Here's how the part is built. I have some questions about the finished solid (model axes, mm). A direction names the side the tool comes from. Give positions to 0.01 mm unless a question says otherwise; leave off trailing zeros. Loops run counter-clockwise (first coordinate to the right, second up) from the corner with the lowest first, then second, coordinate; pieces in that order, holes last. Notation, with made-up numbers: (-2, 68) - (37, 68) arc R19 ccw to (37, 73) - close; hole circle Ø3 at (-38, 7). An arc over 180 degrees is marked (long way). Return JSON: item names as keys, results as strings. Group by question number.
(1) If we section it at D-D (z = 19.5): State how many separate pieces and enclosed holes the cut face has, then the cut area to 3 significant figures.
(2) If we section it at B-B (y = 6.75): Please give me the cut outline in (x, z), then the cut area to 3 significant figures.
(3) If we section it at A-A (x = -11.25): Please give me the cut outline in (y, z) (3 decimals).
(4) I need wall thicknesses on probe 1 along X at (y, z) = (-12, 0) (3 decimals); probe 2 along Y at (x, z) = (-5.25, 6). Which ranges of each line are inside material? Lowest first, please. Write a range as [from, to].
(5) On a 3-axis mill with a long thin cutter (end or side, diameter ignored), from which of +Z, -Z, +X, -X, +Y, -Y can I reach the whole of each face in a straight line? I mean faces 1 (the flat face through (6, -3, 0)), 2 (the flat face through (11, 8.325, 0)), 3 (the flat face through (4.2, -13, 0)), 4 (the flat face through (3, 6, 0)). Say none if no direction works.
(6) If we mould it in two halves opening along X, with no side actions, what happens to faces 5 (the flat face through (-11, -8.325, 0)), 6 (the flat face through (-13, 4.2, 0)), 7 (the flat face through (-6, 3, 0))? For each: released by +X, released by -X, zero draft, split by the parting line, or undercut.
(7) If we section it at C-C (y = 2.5): Please give me the cut outline in (x, z), then the cut area to 3 significant figures.
(8) For P1, Ø5, axis at x = 0, y = 1, coming from the +Z side, with a flat end and sliding along its axis, tell me the tip position at first contact or that it passes through.
```python
from build123d import *

# Parameters (mm, degrees)
BOSS_EXTRUDE1_DEPTH = 30


with BuildPart() as part:
    # Sketch1 → Boss-Extrude1 (new body, symmetric)
    with BuildSketch(Plane.XY):
        with BuildLine():
            Line((-8.325, 12.75), (-4.2, 12.75))
            Line((-4.2, 12.75), (-4.2, 14))
            ThreePointArc((-4.2, 14), (-4.331801948, 14.318198052), (-4.65, 14.45))
            Line((-4.65, 14.45), (-4.7, 14.45))
            Line((-4.7, 14.45), (-4.7, 14.5))
            ThreePointArc((-4.7, 14.5), (-4.831801948, 14.818198052), (-5.15, 14.95))
            Line((-5.15, 14.95), (-13.2, 14.95))
            ThreePointArc((-13.2, 14.95), (-14.437436867, 14.437436867), (-14.95, 13.2))
            Line((-14.95, 13.2), (-14.95, 5.15))
            ThreePointArc((-14.95, 5.15), (-14.818198052, 4.831801948), (-14.5, 4.7))
            Line((-14.5, 4.7), (-14.45, 4.7))
            Line((-14.45, 4.7), (-14.45, 4.65))
            ThreePointArc((-14.45, 4.65), (-14.318198052, 4.331801948), (-14, 4.2))
            Line((-14, 4.2), (-12.75, 4.2))
            Line((-12.75, 4.2), (-12.75, 8.325))
            Line((-12.75, 8.325), (-10.13519336, 8.325))
            Line((-10.13519336, 8.325), (-6, 4.18980664))
            Line((-6, 4.18980664), (-6, 0.875))
            Line((-6, 0.875), (-5.5, 0))
            Line((-5.5, 0), (-6, -0.875))
            Line((-6, -0.875), (-6, -4.18980664))
            Line((-6, -4.18980664), (-10.13519336, -8.325))
            Line((-10.13519336, -8.325), (-12.75, -8.325))
            Line((-12.75, -8.325), (-12.75, -4.2))
            Line((-12.75, -4.2), (-14, -4.2))
            ThreePointArc((-14, -4.2), (-14.318198052, -4.331801948), (-14.45, -4.65))
            Line((-14.45, -4.65), (-14.45, -4.7))
            Line((-14.45, -4.7), (-14.5, -4.7))
            ThreePointArc((-14.5, -4.7), (-14.818198052, -4.831801948), (-14.95, -5.15))
            Line((-14.95, -5.15), (-14.95, -13.2))
            ThreePointArc((-14.95, -13.2), (-14.437436867, -14.437436867), (-13.2, -14.95))
            Line((-13.2, -14.95), (-5.15, -14.95))
            ThreePointArc((-5.15, -14.95), (-4.831801948, -14.818198052), (-4.7, -14.5))
            Line((-4.7, -14.5), (-4.7, -14.45))
            Line((-4.7, -14.45), (-4.65, -14.45))
            ThreePointArc((-4.65, -14.45), (-4.331801948, -14.318198052), (-4.2, -14))
            Line((-4.2, -14), (-4.2, -12.75))
            Line((-4.2, -12.75), (-8.325, -12.75))
            Line((-8.325, -12.75), (-8.325, -10.13519336))
            Line((-8.325, -10.13519336), (-4.18980664, -6))
            Line((-4.18980664, -6), (-0.875, -6))
            Line((-0.875, -6), (0, -5.5))
            Line((0, -5.5), (0.875, -6))
            Line((0.875, -6), (4.18980664, -6))
            Line((4.18980664, -6), (8.325, -10.13519336))
            Line((8.325, -10.13519336), (8.325, -12.75))
            Line((8.325, -12.75), (4.2, -12.75))
            Line((4.2, -12.75), (4.2, -14))
            ThreePointArc((4.2, -14), (4.331801948, -14.318198052), (4.65, -14.45))
            Line((4.65, -14.45), (4.7, -14.45))
            Line((4.7, -14.45), (4.7, -14.5))
            ThreePointArc((4.7, -14.5), (4.831801948, -14.818198052), (5.15, -14.95))
            Line((5.15, -14.95), (13.2, -14.95))
            ThreePointArc((13.2, -14.95), (14.437436867, -14.437436867), (14.95, -13.2))
            Line((14.95, -13.2), (14.95, -5.15))
            ThreePointArc((14.95, -5.15), (14.818198052, -4.831801948), (14.5, -4.7))
            Line((14.5, -4.7), (14.45, -4.7))
            Line((14.45, -4.7), (14.45, -4.65))
            ThreePointArc((14.45, -4.65), (14.318198052, -4.331801948), (14, -4.2))
            Line((14, -4.2), (12.75, -4.2))
            Line((12.75, -4.2), (12.75, -8.325))
            Line((12.75, -8.325), (10.13519336, -8.325))
            Line((10.13519336, -8.325), (6, -4.18980664))
            Line((6, -4.18980664), (6, -0.875))
            Line((6, -0.875), (5.5, 0))
            Line((5.5, 0), (6, 0.875))
            Line((6, 0.875), (6, 4.18980664))
            Line((6, 4.18980664), (10.134787333, 8.324593973))
            Line((10.134787333, 8.324593973), (12.75, 8.324593973))
            Line((12.75, 8.324593973), (12.75, 4.2))
            Line((12.75, 4.2), (14, 4.2))
            ThreePointArc((14, 4.2), (14.318198052, 4.331801948), (14.45, 4.65))
            Line((14.45, 4.65), (14.45, 4.7))
            Line((14.45, 4.7), (14.5, 4.7))
            ThreePointArc((14.5, 4.7), (14.818198052, 4.831801948), (14.95, 5.15))
            Line((14.95, 5.15), (14.95, 13.2))
            ThreePointArc((14.95, 13.2), (14.437436867, 14.437436867), (13.2, 14.95))
            Line((13.2, 14.95), (5.15, 14.95))
            ThreePointArc((5.15, 14.95), (4.831801948, 14.818198052), (4.7, 14.5))
            Line((4.7, 14.5), (4.7, 14.45))
            Line((4.7, 14.45), (4.65, 14.45))
            ThreePointArc((4.65, 14.45), (4.331801948, 14.318198052), (4.2, 14))
            Line((4.2, 14), (4.2, 12.75))
            Line((4.2, 12.75), (8.324593973, 12.75))
            Line((8.324593973, 12.75), (8.324593973, 10.134787333))
            Line((8.324593973, 10.134787333), (4.18980664, 6))
            Line((4.18980664, 6), (0.875, 6))
            Line((0.875, 6), (0, 5.5))
            Line((0, 5.5), (-0.875, 6))
            Line((-0.875, 6), (-4.18980664, 6))
            Line((-4.18980664, 6), (-8.325, 10.13519336))
            Line((-8.325, 10.13519336), (-8.325, 12.75))
        make_face()
        with BuildLine():
            Line((-4.478803313, -3.194699355), (-3.226318161, -1.597144679))
            ThreePointArc((-3.226318161, -1.597144679), (-3.6, 0), (-3.226318161, 1.597144679))
            Line((-3.226318161, 1.597144679), (-4.478803313, 3.194699355))
            ThreePointArc((-4.478803313, 3.194699355), (-3.890101739, 3.890101739), (-3.194699355, 4.478803313))
            Line((-3.194699355, 4.478803313), (-1.597144679, 3.226318161))
            ThreePointArc((-1.597144679, 3.226318161), (0, 3.6), (1.597144679, 3.226318161))
            Line((1.597144679, 3.226318161), (3.194699355, 4.478803313))
            ThreePointArc((3.194699355, 4.478803313), (3.890101739, 3.890101739), (4.478803313, 3.194699355))
            Line((4.478803313, 3.194699355), (3.226318161, 1.597144679))
            ThreePointArc((3.226318161, 1.597144679), (3.6, 0), (3.226318161, -1.597144679))
            Line((3.226318161, -1.597144679), (4.478803313, -3.194699355))
            ThreePointArc((4.478803313, -3.194699355), (3.890101739, -3.890101739), (3.194699355, -4.478803313))
            Line((3.194699355, -4.478803313), (1.597144679, -3.226318161))
            ThreePointArc((1.597144679, -3.226318161), (0, -3.6), (-1.597144679, -3.226318161))
            Line((-1.597144679, -3.226318161), (-3.194699355, -4.478803313))
            ThreePointArc((-3.194699355, -4.478803313), (-3.890101739, -3.890101739), (-4.478803313, -3.194699355))
        make_face(mode=Mode.SUBTRACT)
        with BuildLine():
            Line((-13.65, -12.65), (-13.65, -10.5))
            ThreePointArc((-13.65, -10.5), (-13.357106781, -9.792893219), (-12.65, -9.5))
            Line((-12.65, -9.5), (-10.5, -9.5))
            ThreePointArc((-10.5, -9.5), (-9.792893219, -9.792893219), (-9.5, -10.5))
            Line((-9.5, -10.5), (-9.5, -12.65))
            ThreePointArc((-9.5, -12.65), (-9.792893219, -13.357106781), (-10.5, -13.65))
            Line((-10.5, -13.65), (-12.65, -13.65))
            ThreePointArc((-12.65, -13.65), (-13.357106781, -13.357106781), (-13.65, -12.65))
        make_face(mode=Mode.SUBTRACT)
        with BuildLine():
            Line((9.5, 10.5), (9.5, 12.65))
            ThreePointArc((9.5, 12.65), (9.792893219, 13.357106781), (10.5, 13.65))
            Line((10.5, 13.65), (12.65, 13.65))
            ThreePointArc((12.65, 13.65), (13.357106781, 13.357106781), (13.65, 12.65))
            Line((13.65, 12.65), (13.65, 10.5))
            ThreePointArc((13.65, 10.5), (13.357106781, 9.792893219), (12.65, 9.5))
            Line((12.65, 9.5), (10.5, 9.5))
            ThreePointArc((10.5, 9.5), (9.792893219, 9.792893219), (9.5, 10.5))
        make_face(mode=Mode.SUBTRACT)
        with BuildLine():
            Line((-13.65, 10.5), (-13.65, 12.65))
            ThreePointArc((-13.65, 12.65), (-13.357106781, 13.357106781), (-12.65, 13.65))
            Line((-12.65, 13.65), (-10.5, 13.65))
            ThreePointArc((-10.5, 13.65), (-9.792893219, 13.357106781), (-9.5, 12.65))
            Line((-9.5, 12.65), (-9.5, 10.5))
            ThreePointArc((-9.5, 10.5), (-9.792893219, 9.792893219), (-10.5, 9.5))
            Line((-10.5, 9.5), (-12.65, 9.5))
            ThreePointArc((-12.65, 9.5), (-13.357106781, 9.792893219), (-13.65, 10.5))
        make_face(mode=Mode.SUBTRACT)
        with BuildLine():
            Line((10.5, -9.5), (12.65, -9.5))
            ThreePointArc((12.65, -9.5), (13.357106781, -9.792893219), (13.65, -10.5))
            Line((13.65, -10.5), (13.65, -12.65))
            ThreePointArc((13.65, -12.65), (13.357106781, -13.357106781), (12.65, -13.65))
            Line((12.65, -13.65), (10.5, -13.65))
            ThreePointArc((10.5, -13.65), (9.792893219, -13.357106781), (9.5, -12.65))
            Line((9.5, -12.65), (9.5, -10.5))
            ThreePointArc((9.5, -10.5), (9.792893219, -9.792893219), (10.5, -9.5))
        make_face(mode=Mode.SUBTRACT)
    extrude(amount=BOSS_EXTRUDE1_DEPTH, both=True)


solid = part.part
```
Values:
{
 "1": {"separate pieces": "1", "enclosed holes": "5", "area": "310 mm2"},
 "2": {"outline": "(-14.95, -30) - (-12.75, -30) - (-12.75, 30) - (-14.95, 30) - close; (-8.56, -30) - (-4.94, -30) - (-4.94, 30) - (-8.56, 30) - close; (4.94, -30) - (8.56, -30) - (8.56, 30) - (4.94, 30) - close; (12.75, -30) - (14.95, -30) - (14.95, 30) - (12.75, 30) - close", "area": "698 mm2"},
 "3": {"outline": "(-14.95, -30) - (-13.65, -30) - (-13.65, 30) - (-14.95, 30) - close; (-9.5, -30) - (-8.325, -30) - (-8.325, 30) - (-9.5, 30) - close; (8.325, -30) - (9.5, -30) - (9.5, 30) - (8.325, 30) - close; (13.65, -30) - (14.95, -30) - (14.95, 30) - (13.65, 30) - close"},
 "4": {"probe 1": "[-14.95, -13.65], [-9.5, -8.325], [8.325, 9.5], [13.65, 14.95]", "probe 2": "[-14.95, -12.75], [-7.06, 7.06], [12.75, 14.95]"},
 "5": {"face 1": "+Z, -Z, +X", "face 2": "+Z, -Z", "face 3": "+Z, -Z, -Y", "face 4": "+Z, -Z, +Y"},
 "6": {"face 5": "undercut", "face 6": "zero draft", "face 7": "released by -X"},
 "7": {"outline": "(-6, -30) - (-3.93, -30) - (-3.93, 30) - (-6, 30) - close; (3.93, -30) - (6, -30) - (6, 30) - (3.93, 30) - close", "area": "248 mm2"},
 "8": {"P1": "through"}
}
